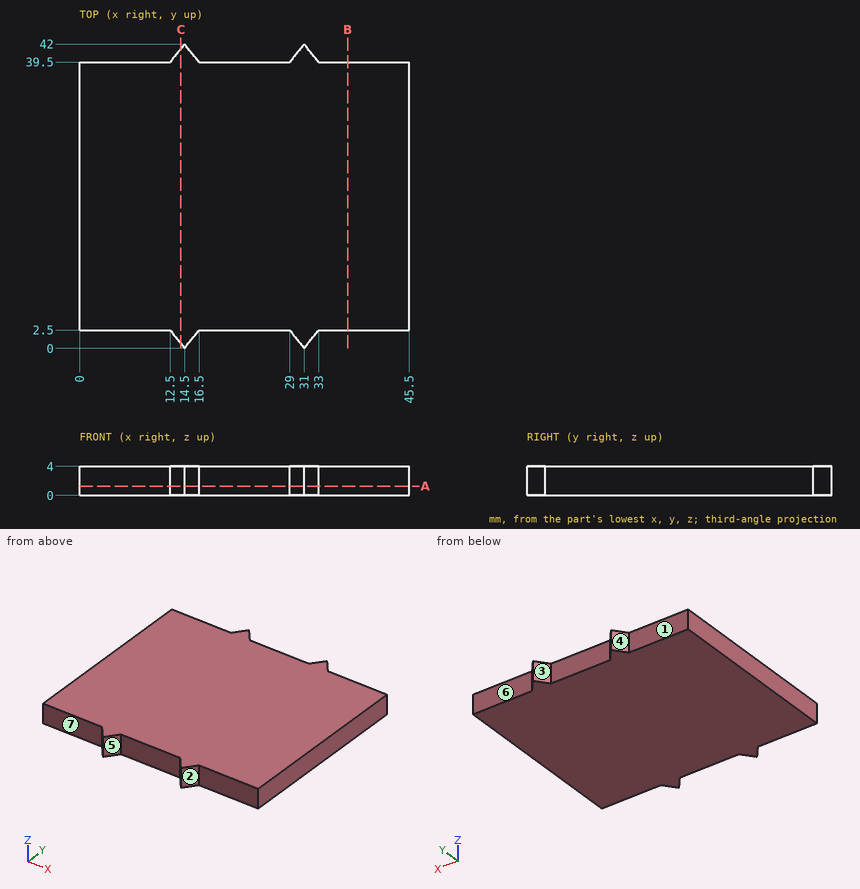
Geometry: see drawing. Coordinates: mm, zero at the bounding-box minimum. A direction names the side the tool comes from. Give positions to 0.01 mm unless a question says otherwise; leave off trailing zeros. Write each loop counter-clockwise with the first axis right and the second up, starting at its lowest first coordinate (ties: lowest second). Pieces come first, ordered by that corner, then holes. Notation, with made-up numbers: M 35,85 L 70,85 A28 cw 70,113 Z; hole C 29.5,24.5 d1. An arc over 180 degrees is marked long. Answer as a JSON object with one key per item and string values.
Q1. Mould query, pull axis X, two halves, no side actions, for the marked faces 1, 2, 3 and 4. Classes: +X half, -X half, draft (parallel to the pull), parting line (faces both ways), or undercut.
Geometry check:
{"face 1": "draft", "face 2": "+X half", "face 3": "undercut", "face 4": "-X half"}
Q2. Cut plane C-C, the plane x = 14. Return the cut outline in (y, z) (3 decimals), then the cut area to 3 significant figures.
Geometry check:
{"outline": "M 0.625,0 L 41.375,0 L 41.375,4 L 0.625,4 Z", "area": "163 mm^2"}
Q3. Cut plane B-B, the plane x = 37. Return the cut outline in (y, z), then the cut area to 3 significant figures.
Geometry check:
{"outline": "M 2.5,0 L 39.5,0 L 39.5,4 L 2.5,4 Z", "area": "148 mm^2"}
Q4. Cut plane A-A, the plane z = 1.25. Return the cut outline in (x, y), then the cut area to 3 significant figures.
Geometry check:
{"outline": "M 0,2.5 L 12.5,2.5 L 14.5,0 L 16.5,2.5 L 29,2.5 L 31,0 L 33,2.5 L 45.5,2.5 L 45.5,39.5 L 33,39.5 L 31,42 L 29,39.5 L 16.5,39.5 L 14.5,42 L 12.5,39.5 L 0,39.5 Z", "area": "1,700 mm^2"}
Q5. Access query for the marked faces 5, 6 and 7. Directions: +Z, -Z, +X, -X, +Y, -Y. A direction counts if a zero-diameter tool reaches every point of the face in a straight line with its end or side. Return the directions, or none.
Geometry check:
{"face 5": "+Z, -Z, -Y", "face 6": "+Z, -Z, +X, +Y", "face 7": "+Z, -Z, -X, -Y"}
Q6. Contact query for flat-ended pins moving along their axis: P1, Ø1.2, axis at x = 22.5, z = 2, coming from the +Y side; P2, Ø1.2, axis at x = 42, z = 2, coming from the -Y side. Output: stop coordinate, or through.
Geometry check:
{"P1": "stops at y = 39.5", "P2": "stops at y = 2.5"}
Q7. Ray query, line 1 along Y through (x, z) = (5, 1.5); line 2 along Y through (x, z) = (13, 3.35) (3 decimals). Return the intervals inside material, ascending.
Geometry check:
{"line 1": "y = 2.5 to 39.5", "line 2": "y = 1.875 to 40.125"}
